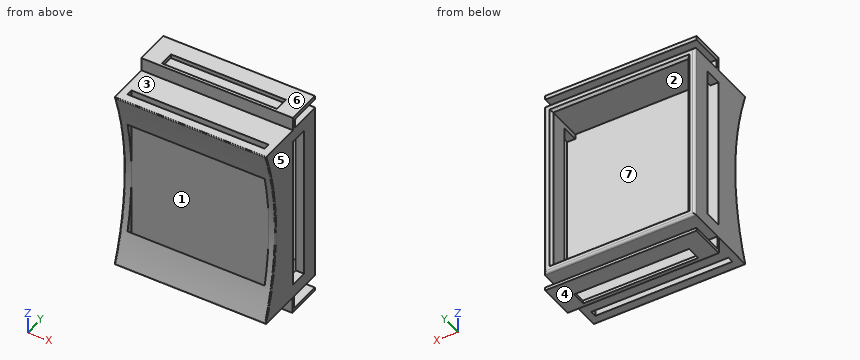
Autodesk Inventor part; units mm, degrees
ref_plane "Work Plane1" through (0, 15.24, 0) normal (0, 1, 0) x (1, 0, 0)
ref_plane "Work Plane2" through (18.6648, 4.7106, -31.4933) normal (0, 0, -1) x (-1, 0, 0)
ref_plane "YZ Plane" through (0, 0, 0) normal (1, 0, 0) x (0, 1, 0)
sketch "Sketch1" plane through (0, 0, 0) normal (0, 1, 0) x (-1, 0, 0)
  line L0 (28.4151, 25.1868) -> (-18.6648, 25.1868)
  line L1 (-18.6648, 25.1868) -> (-18.6648, -31.4933)
  line L2 (-18.6648, -31.4933) -> (28.4151, -31.4933)
  line L3 (28.4151, -31.4933) -> (28.4151, 25.1868)
  dimension "d1" = 47.0799
  dimension "d2" = 56.6801
extrude "Extrusion1" add sketch "Sketch1" along normal blind 15.24
sketch "Sketch3" plane through (18.6648, 0, 25.1868) normal (1, 0, 0) x (0, 0, -1)
  line L0 (0, 15.24) -> (56.6801, 15.24)
  line L1 (0, 0) -> (0, 15.24)
  line L2 (0, 4.3509) -> (0, 0)
  line L3 (0, 0) -> (56.6801, 0)
  line L4 (0, 0) -> (56.6801, 0)
  line L5 (56.6801, 0) -> (56.6801, 4.3509)
  line L6 (56.6801, 0) -> (56.6801, 15.24)
  arc A0 (56.6801, 4.3509) -> (0, 4.3509) centre (28.3401, -74.9624) ccw
  point P0 (25.1868, 0)
extrude "Extrusion2" cut sketch "Sketch3" against normal through all contours A0 L5 L3 L1
fillet "Fillet1" radius 0.254 4 edges at (18.6648, 9.262, -3.1532) (-4.8752, 4.3509, -31.4933) (-28.4151, 9.262, -3.1532) (-4.8752, 4.3509, 25.1868)
sketch "Sketch4" plane through (0, 15.24, 0) normal (0, 1, 0) x (1, 0, 0)
  point P0 (0, 0)
ref_plane "Work Plane1" through (0, 15.24, 0) normal (0, 1, 0) x (1, 0, 0)
sketch "Sketch8" plane through (0, 15.24, 0) normal (0, 1, 0) x (1, 0, 0)
  line L0 (-28.4151, -25.1868) -> (18.6648, -25.1868)
  line L1 (-28.4151, -25.1868) -> (18.6648, -25.1868)
  line L2 (18.6648, -25.1868) -> (18.6648, 31.4933)
  line L3 (18.6648, 31.4933) -> (-28.4151, 31.4933)
  line L4 (-28.4151, 31.4933) -> (-28.4151, -25.1868)
  point P0 (0, 0)
extrude "Extrusion5" add sketch "Sketch8" along normal blind 14.19
sketch "Sketch9" plane through (0, 29.43, 0) normal (0, 1, 0) x (1, 0, 0)
  line L0 (-28.4151, -25.1868) -> (-28.4151, -25.1722)
  line L1 (18.6648, 31.4933) -> (18.6648, 31.4787)
  line L2 (18.6648, -25.1722) -> (18.6648, -25.1868)
  line L3 (-28.4151, 31.4933) -> (18.6648, 31.4933)
  line L4 (-25.8751, -22.6468) -> (16.1248, -22.6468)
  line L5 (16.1248, -22.6468) -> (16.1248, 28.9532)
  line L6 (16.1248, 28.9532) -> (-25.8751, 28.9532)
  line L7 (-25.8751, 28.9532) -> (-25.8751, -22.6468)
  line L8 (-25.8751, -22.6468) -> (16.1248, 28.9532) construction
  line L9 (16.1248, -22.6468) -> (-25.8751, 28.9532) construction
  point P0 (0, 0)
  point P1 (-4.8752, 3.1532)
  dimension "d30" = 41.9999
  dimension "d31" = 51.6
extrude "Extrusion6" cut sketch "Sketch9" against normal blind 11.65
fillet "Fillet2" radius 0.762 4 edges at (-28.4151, 29.43, -3.1532) (-4.8752, 29.43, -31.4933) (18.6648, 29.43, -3.1532) (-4.8752, 29.43, 25.1868)
chamfer "Chamfer3" distance 0.762 angle 45 4 edges at (-4.8752, 29.43, 22.6468) (16.1248, 29.43, -3.1532) (-4.8752, 29.43, -28.9532) (-25.8751, 29.43, -3.1532)
sketch "Sketch10" plane through (18.6648, -74.9624, -3.1532) normal (1, 0, 0) x (0, 0, -1)
  arc A0 (28.3255, 79.5882) -> (-28.3255, 79.5882) centre (0, 0) ccw
  line L0 (28.34, 79.673) -> (28.34, 103.6304)
  line L1 (-28.3255, 79.5882) -> (28.34, 79.5882)
  line L2 (28.34, 79.5882) -> (28.34, 83.3201)
  line L3 (28.34, 83.3201) -> (-28.3255, 83.3201)
  line L4 (-28.3255, 83.3201) -> (-28.3255, 79.5882)
  point P0 (-3.1532, 74.9624)
ref_plane "Work Plane2" through (18.6648, 4.7106, -31.4933) normal (0, 0, -1) x (-1, 0, 0)
sketch "Sketch11" plane through (18.6648, 4.7106, -31.4933) normal (0, 0, -1) x (-1, 0, 0)
  line L0 (0, 4.8055) -> (0, -0.0848)
  line L1 (47.0799, -0.0848) -> (47.0799, 4.8055)
  line L2 (0, 4.8055) -> (47.0799, 4.8055)
  line L3 (47.0799, 4.8055) -> (47.0799, -0.0848)
  line L4 (47.0799, -0.0848) -> (0, -0.0848)
  line L5 (0, -0.0848) -> (0, 4.8055)
  line L6 (0.254, 4.5515) -> (46.8259, 4.5515)
  line L7 (2.1582, 4.5515) -> (44.8203, 4.5515)
  line L8 (44.8203, 4.5515) -> (44.8203, 2.5848)
  line L9 (44.8203, 2.5848) -> (2.1582, 2.5848)
  line L10 (2.1582, 2.5848) -> (2.1582, 4.5515)
  point P0 (18.6648, -4.7106)
extrude "Extrusion7" cut sketch "Sketch11" against normal through all contours L6 L8 L9 L10
sketch "Sketch15" plane through (18.6648, -74.9624, -3.1532) normal (1, 0, 0) x (0, 0, -1)
  line L0 (-25.8, 92.7424) -> (25.8, 92.7424)
  line L1 (-24.298, 98.2163) -> (24.0484, 98.2163)
  line L2 (24.0484, 98.2163) -> (24.0484, 92.7424)
  line L3 (24.0484, 92.7424) -> (-24.298, 92.7424)
  line L4 (-24.298, 92.7424) -> (-24.298, 98.2163)
  point P0 (-3.1532, 74.9624)
  point P1 (-24.298, 92.7424)
extrude "Extrusion8" cut sketch "Sketch15" against normal through all
sketch "Sketch16" plane through (-28.4151, -74.9624, -3.1532) normal (-1, 0, 0) x (0, 0, 1)
  line L0 (28.34, 79.673) -> (28.34, 103.6304)
  line L1 (28.34, 92.7388) -> (32.5027, 92.7388)
  line L2 (32.5027, 92.7388) -> (32.5027, 103.6304)
  line L3 (32.5027, 103.6304) -> (28.34, 103.6304)
  line L4 (28.34, 103.6304) -> (28.34, 92.7388)
  point P0 (3.1532, 74.9624)
extrude "Extrusion9" add sketch "Sketch16" against normal blind 47.0799
sketch "Sketch17" plane through (-28.4151, -74.9624, -3.1532) normal (-1, 0, 0) x (0, 0, 1)
  line L0 (32.5027, 103.6304) -> (28.34, 103.6304)
  line L1 (28.34, 103.6304) -> (31.2211, 103.6304)
  line L2 (31.2211, 103.6304) -> (31.2211, 93.7101)
  line L3 (31.2211, 93.7101) -> (28.34, 93.7101)
  line L4 (28.34, 93.7101) -> (28.34, 103.6304)
  point P0 (3.1532, 74.9624)
  point P1 (31.2211, 103.6304)
extrude "Extrusion10" cut sketch "Sketch17" against normal blind 47.0799
sketch "Sketch18" plane through (18.6648, -74.9624, -3.1532) normal (1, 0, 0) x (0, 0, -1)
  line L0 (28.34, 79.673) -> (28.34, 103.6304)
  line L1 (28.34, 103.6304) -> (33.459, 103.6304)
  line L2 (33.459, 103.6304) -> (33.459, 92.5316)
  line L3 (33.459, 92.5316) -> (28.34, 92.5316)
  line L4 (28.34, 92.5316) -> (28.34, 103.6304)
  point P0 (-3.1532, 74.9624)
extrude "Extrusion11" add sketch "Sketch18" against normal blind 47.0799
sketch "Sketch19" plane through (18.6648, -74.9624, -3.1532) normal (1, 0, 0) x (0, 0, -1)
  line L0 (28.34, 103.6304) -> (32.4698, 103.6304)
  line L1 (32.4698, 103.6304) -> (32.4698, 93.2696)
  line L2 (32.4698, 93.2696) -> (28.34, 93.2696)
  line L3 (28.34, 93.2696) -> (28.34, 103.6304)
  point P0 (-3.1532, 74.9624)
extrude "Extrusion12" cut sketch "Sketch19" against normal blind 47.0799
sketch "Sketch20" plane through (18.6648, 17.5691, -36.6123) normal (0, 0, -1) x (-1, 0, 0)
  line L0 (47.0799, 1.1785) -> (0, 1.1785)
  line L1 (5.5367, 5.6549) -> (41.372, 5.6549)
  line L2 (41.372, 5.6549) -> (41.372, 1.1785)
  line L3 (41.372, 1.1785) -> (5.5367, 1.1785)
  line L4 (5.5367, 1.1785) -> (5.5367, 5.6549)
  point P0 (18.6648, -17.5691)
  point P1 (5.5367, 1.1785)
extrude "Extrusion13" cut sketch "Sketch20" against normal blind 1.778
sketch "Sketch21" plane through (-28.4151, 17.7764, 29.3495) normal (0, 0, 1) x (1, 0, 0)
  line L0 (5.7079, 0.9713) -> (5.7079, 5.4477)
  line L1 (41.5432, 0.9713) -> (5.7079, 0.9713)
  line L2 (5.7079, 5.4477) -> (41.5432, 5.4477)
  line L3 (41.5432, 5.4477) -> (41.5432, 0.9713)
  line L4 (41.5432, 0.9713) -> (5.7079, 0.9713)
  line L5 (5.7079, 0.9713) -> (5.7079, 5.4477)
  point P0 (28.4151, -17.7764)
extrude "Extrusion14" cut sketch "Sketch21" against normal blind 1.778
properties part number "wear1"
Check sheet for the modelled part. Datum: model origin and axes. Units: mm. Face numbers are marked on the shaded views. A direction names the side the tool comes from. Give positions to 0.01 mm unless a question says otherwise; leave off trailing zeros. Use one line per item in the form item = value.
(1) Section check A-A on x = -24. State how many separate pieces and enclosed holes the cut face has, plus the area to 3 significant figures.
Answer block:
separate_pieces = 3
enclosed_holes = 0
area = 600 mm2
(2) Draft check along Z on the marked faces 5, 6 and 7. Enter one of: pulls with the +Z half, pulls with the -Z half, needs draft (parallel to the pull), parting line crosses it, or undercut.
Answer block:
face_5 = needs draft
face_6 = pulls with the +Z half
face_7 = undercut
(3) Material ranges on line 1 along X through (y, z) = (23.5, 11.5); line 2 along Z through (x, y) = (-18, 26.75); line 3 along Y through (x, z) = (-19.5, -10), recorded low to high.
Answer block:
line_1 = -28.42 to -25.88, 16.12 to 18.66
line_2 = -36.61 to -35.62, -31.49 to -28.95, 22.65 to 25.19, 28.07 to 29.35
line_3 = 9.26 to 17.78
(4) Tool access check on the marked faces 1, 2, 3 and 4. Record the directions out of +Z, -Z, +X, -X, +Y, -Y that give a thin tool (end or side, any length) a straight path to the whole face; none if there is none.
Answer block:
face_1 = +Z, -Z
face_2 = +Y
face_3 = +Z, +X, -X, -Y
face_4 = -Z, +X, -X, +Y, -Y
(5) Depth check by flat-ended pin: P1, Ø1, axis at x = -15, z = -2, coming from the -Y side; P2, Ø1.5, axis at x = 7, z = -22.5, coming from the +Y side; P3, Ø1.4, axis at x = -14, z = 28.5, coming from the +Y side. Enter the tip coordinate at first touch or a pass-through.
Answer block:
P1 = 9.26
P2 = 17.78
P3 = 28.67
